Input: part model. Units: mm. Frame: model coordinates. Round coordinates to 2 decimals unless told otherwise and drop trailing zeros. Loops run counter-clockwise (first coordinate to the right, second up) from the corner with the lowest first, then second, coordinate; pieces in that order, holes last. Notation, with made-up numbers: M -8,8.25 L 17,8.25 A25 ccw 17,22.25 Z; hole C 81.5,43 d11. An arc over 180 degrees is marked long. Put each result on its own line as item: value. Start each with the question number.
1) Section A-A on x = 12.7. Output: boundary loops of the cut face in (y, z) (3 decimals), plus the area to 3 significant figures.
2) Section D-D on z = 1.7. Output: boundary loops of the cut face in (x, y) (3 decimals).
3) Line query: probe 1 along Y at (x, z) = (-12.7, 1.4) (3 decimals); probe 2 along Y at (x, z) = (36.5, 2.05); probe 3 along X at (y, z) = (39, 0.9). Output: solid intervals per line, ascending.
4) Section B-B on x = 38.1. Output: boundary loops of the cut face in (y, z) (3 decimals).
5) Pin query (flat end, axial travel): pin 1 (0.6 mm diameter, centred on y = 29, z = 2, fed in from -X); pin 2 (5 mm diameter, centred on x = 38.1, y = 12.7, fed in from -Z); pin 3 (8.5 mm diameter, centred on x = 12.7, y = 12.7, fed in from -Z); pin 4 (1.6 mm diameter, centred on x = -11.5, z = 2, fed in from +Y). Return the tip coordinate at first contact, or that it passes through.
6) Section C-C on y = 12.7. Output: boundary loops of the cut face in (x, z) (3 decimals), plus the area to 3 significant figures.
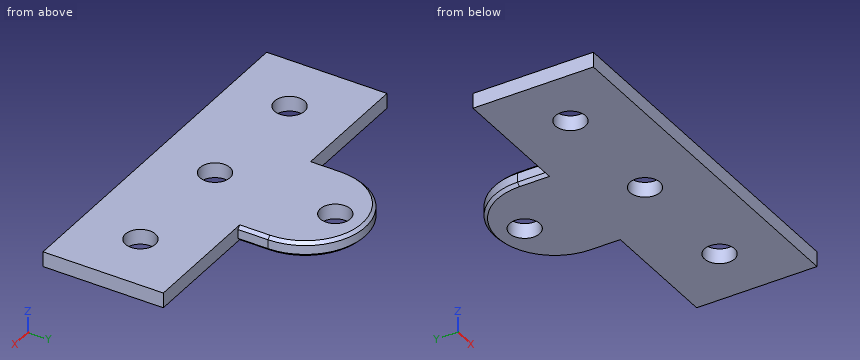
from build123d import *

# Parameters (mm, degrees)
SKETCH1_R           = 3.175
BOSS_EXTRUDE1_DEPTH = 3.175
CHAMFER2_SIZE       = 0.635


with BuildPart() as part:
    # Sketch1 → Boss-Extrude1 (new body)
    with BuildSketch(Plane.XY):
        with BuildLine():
            Line((0, 0), (25.4, 0))
            Line((25.4, 0), (50.8, 0))
            Line((50.8, 0), (50.8, 25.4))
            Line((50.8, 25.4), (25.4, 25.4))
            Line((25.4, 25.4), (25.4, 31.75))
            ThreePointArc((25.4, 31.75), (12.7, 44.45), (0, 31.75))
            Line((0, 31.75), (0, 25.4))
            Line((0, 25.4), (-25.4, 25.4))
            Line((-25.4, 25.4), (-25.4, 0))
            Line((-25.4, 0), (0, 0))
        make_face()
        with Locations((12.7, 38.1)):
            Circle(SKETCH1_R, mode=Mode.SUBTRACT)
        with Locations((12.7, 12.7)):
            Circle(SKETCH1_R, mode=Mode.SUBTRACT)
        with Locations((38.1, 12.7)):
            Circle(SKETCH1_R, mode=Mode.SUBTRACT)
        with Locations((-12.7, 12.7)):
            Circle(SKETCH1_R, mode=Mode.SUBTRACT)
    extrude(amount=BOSS_EXTRUDE1_DEPTH)

    # Chamfer2
    chamfer2_edges = [part.edges().sort_by_distance(p)[0] for p in [
        (0, 28.575, 0),
        (12.7, 44.45, 0),
        (25.4, 28.575, 0),
        (25.4, 28.575, 3.175),
        (12.7, 44.45, 3.175),
        (0, 28.575, 3.175),
    ]]
    chamfer(chamfer2_edges, length=CHAMFER2_SIZE)


solid = part.part
Geometry results:
1. outline: M 0,0 L 9.525,0 L 9.525,3.175 L 0,3.175 Z; M 15.875,0 L 34.925,0 L 34.925,3.175 L 15.875,3.175 Z; M 41.275,0 L 43.815,0 L 44.45,0.635 L 44.45,2.54 L 43.815,3.175 L 41.275,3.175 Z
1. area: 100 mm²
2. outline: M -25.4,0 L 50.8,0 L 50.8,25.4 L 25.4,25.4 L 25.4,31.75 A12.7 ccw 0,31.75 L 0,25.4 L -25.4,25.4 Z; hole C -12.7,12.7 d6.35; hole C 12.7,12.7 d6.35; hole C 12.7,38.1 d6.35; hole C 38.1,12.7 d6.35
3. probe 1: y = 0 to 9.525, 15.875 to 25.4
3. probe 2: y = 0 to 9.96, 15.44 to 25.4
3. probe 3: x = 2.27 to 9.66, 15.74 to 23.13
4. outline: M 0,0 L 9.525,0 L 9.525,3.175 L 0,3.175 Z; M 15.875,0 L 25.4,0 L 25.4,3.175 L 15.875,3.175 Z
5. pin 1: stops at x = 0
5. pin 2: passes through
5. pin 3: stops at z = 0
5. pin 4: stops at y = 25.4
6. outline: M -25.4,0 L -15.875,0 L -15.875,3.175 L -25.4,3.175 Z; M -9.525,0 L 9.525,0 L 9.525,3.175 L -9.525,3.175 Z; M 15.875,0 L 34.925,0 L 34.925,3.175 L 15.875,3.175 Z; M 41.275,0 L 50.8,0 L 50.8,3.175 L 41.275,3.175 Z
6. area: 181 mm²
